```python
from build123d import *

# Parameters (mm, degrees)
SKETCH1_W           = 330.2
SKETCH1_H           = 508
BOSS_EXTRUDE1_DEPTH = 25.4
SKETCH2_R           = 25.4
BOSS_EXTRUDE2_DEPTH = 12.7


with BuildPart() as part:
    # Sketch1 → Boss-Extrude1 (new body)
    with BuildSketch(Plane(origin=(0, 0, 0), x_dir=(1, 0, 0), z_dir=(0, 1, 0))):
        with Locations((58.531016631, -24.295652174)):
            Rectangle(SKETCH1_W, SKETCH1_H)
    extrude(amount=BOSS_EXTRUDE1_DEPTH)

    # Sketch2 → Boss-Extrude2 (add)
    with BuildSketch(Plane(origin=(0, 25.4, 0), x_dir=(1, 0, 0), z_dir=(0, 1, 0))):
        with Locations((-24.018983369, 102.704347826)):
            Circle(SKETCH2_R)
        with Locations((141.081016631, 102.704347826)):
            Circle(SKETCH2_R)
        with Locations((141.081016631, -151.295652174)):
            Circle(SKETCH2_R)
        with Locations((-24.018983369, -151.295652174)):
            Circle(SKETCH2_R)
    extrude(amount=BOSS_EXTRUDE2_DEPTH)


solid = part.part
```
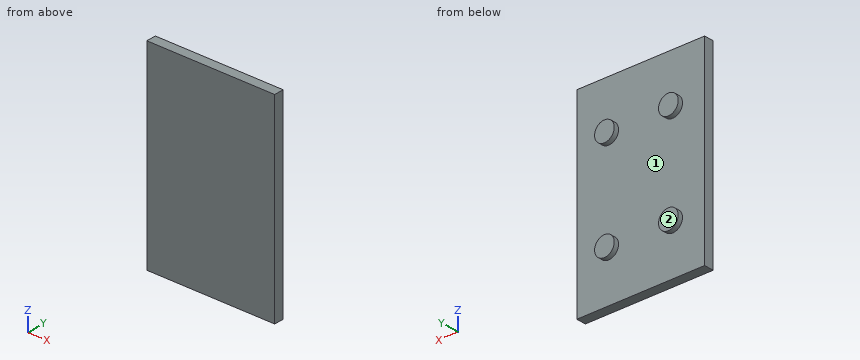
Work out the finished part from the listing and answer in its coordinate system (mm). Face numbers are marked on the shaded views. A direction names the side the tool comes from. Give positions to 0.01 mm unless a question says otherwise; leave off trailing zeros. Loops run counter-clockwise (first coordinate to the right, second up) from the corner with the lowest first, then second, coordinate; pieces in that order, holes last. Notation, with made-up numbers: (65.25, -25.75) -> (83.25, -25.75) arc R27 cw to (83.25, 8.25) -> close; hole circle Ø2 at (46, 4). An arc over 180 degrees is marked (long way). Write item = value, one per line. Start each with the question number.
(1) Find the intervals of material crossed by probe 1 along Y at (x, z) = (-89, 108); probe 2 along Z at (x, y) = (155, 30.5); probe 3 along Z at (x, y) = (-32.5, 29), in increasing order. Write a range as from..to.
(2) Given pin 1 Ø10 at (x, z) = (56, 108.5) entering from +Y; pin 2 Ø5 at (y, z) = (33.5, 142) entering from -X, each flat-ended and moving along its own axis, determine where each tip first touches the part or whether it passes through.
(3) Find section B-B on y = 32. Give the vertices of the cut face in (x, z).
(4) Which of the six approach directions +Z, -Z, +X, -X, +Y, -Y give full straight-line access (tool end or side, diameter ignored) to the marked faces 1 and 2?
(5) Find section A-A on z = -16. Give the vertices of the cut face in (x, y).
(6) Find section C-C on x = 55. Give the vertices of the cut face in (y, z).
From the geometry:
q1.probe_1 = 0..25.4
q1.probe_2 = -123.95..-81.46, 130.05..172.54
q1.probe_3 = -126.65..-78.76, 127.35..175.24
q2.pin_1 = 25.4
q2.pin_2 = -48.49
q3.outline = circle Ø50.8 at (-24.02, -102.7); circle Ø50.8 at (-24.02, 151.3); circle Ø50.8 at (141.08, -102.7); circle Ø50.8 at (141.08, 151.3)
q4.face_1 = +Y
q4.face_2 = +Z, -Z, +X, -X, +Y
q5.outline = (-106.57, 0) -> (223.63, 0) -> (223.63, 25.4) -> (-106.57, 25.4) -> close
q6.outline = (0, -229.7) -> (25.4, -229.7) -> (25.4, 278.3) -> (0, 278.3) -> close
